The drawing under review shows one solid part. Ordinate dimensions are in mm from its lowest x, y, z. A direction names the side the tool comes from. Coordinates: 2 decimals unless noted, no trailing zeros. Order: outer loops, then holes, each group sorted by start corner. A loop starts at its lowest first (then second) coordinate and runs counter-clockwise, first axis right, second up. Notation, with made-up numbers: M 47.25,14.5 L 100.25,14.5 A22 cw 100.25,34.5 Z; hole C 20.25,-27.5 d4. An arc over 180 degrees is marked long. Answer as a JSON object with one key per item and string values.
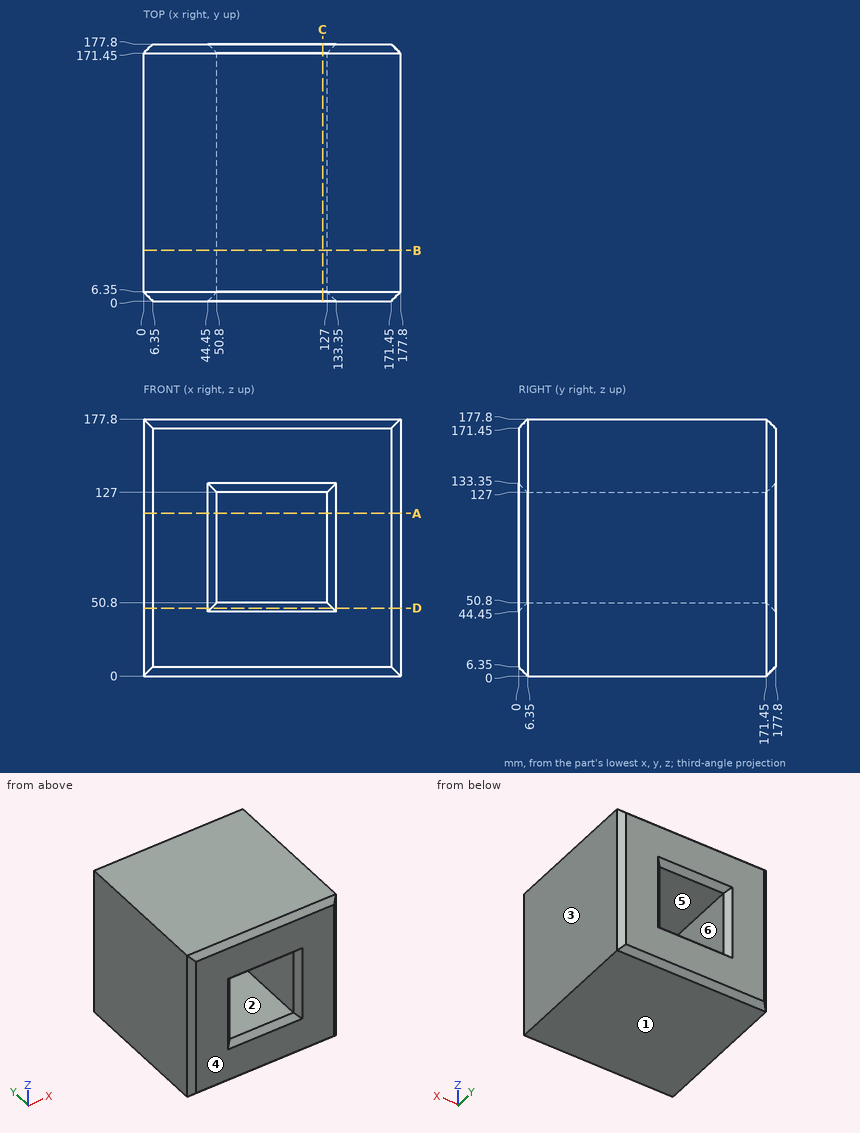
1) Add section D-D (z = 47). State the section outline as (x, y) points, and give its area (3 significant figures).
Taken from the geometry:
{"outline": "M 0,6.35 L 6.35,0 L 44.45,0 L 47,2.55 L 130.8,2.55 L 133.35,0 L 171.45,0 L 177.8,6.35 L 177.8,171.45 L 171.45,177.8 L 133.35,177.8 L 130.8,175.25 L 47,175.25 L 44.45,177.8 L 6.35,177.8 L 0,171.45 Z", "area": "31,100 mm2"}
2) Add section B-B (y = 35). State the section outline as (x, z) points, and give its area (3 significant figures).
Taken from the geometry:
{"outline": "M 0,0 L 177.8,0 L 177.8,177.8 L 0,177.8 Z; hole M 50.8,50.8 L 127,50.8 L 127,127 L 50.8,127 Z", "area": "25,800 mm2"}
3) To check wall thickness, follow L1, parallel to X at y = 89.5, z = 60.5; L2, parallel to Y at x = 46, z = 51. State the ranges of each line that lie inside material, in increasing order.
Taken from the geometry:
{"L1": "x = 0 to 50.8, 127 to 177.8", "L2": "y = 1.55 to 176.25"}
4) Insertion check: pin 1 Ø2 at (x, z) = (66, 127.5) entering from -Y; pin 2 Ø3 at (x, z) = (117, 130) entering from +Y. Each pin has a flat end and moves straight along its axis. Give the tip position at first contact, or say it passes through.
Taken from the geometry:
{"pin 1": "stops at y = 4.85", "pin 2": "stops at y = 175.95"}
5) Add section A-A (z = 112.5). State the section outline as (x, y) points, and give its area (3 significant figures).
Taken from the geometry:
{"outline": "M 0,6.35 L 6.35,0 L 44.45,0 L 50.8,6.35 L 50.8,171.45 L 44.45,177.8 L 6.35,177.8 L 0,171.45 Z; M 127,6.35 L 133.35,0 L 171.45,0 L 177.8,6.35 L 177.8,171.45 L 171.45,177.8 L 133.35,177.8 L 127,171.45 Z", "area": "17,900 mm2"}
6) Tool access review of the marked faces 1 and 2: name each direction out of +Z, -Z, +X, -X, +Y, -Y from which nothing blocks a thin tool from reaching the whole face with its end or side.
Taken from the geometry:
{"face 1": "-Z, +X, -X, +Y, -Y", "face 2": "+Y, -Y"}
7) Mouldability with a two-part tool opening along X and no side actions: class the marked faces 3, 4, 5 and 6 as released by +X, released by -X, zero draft, split by the parting line, or undercut.
Taken from the geometry:
{"face 3": "released by +X", "face 4": "zero draft", "face 5": "undercut", "face 6": "undercut"}
8) Add section C-C (x = 124). State the section outline as (y, z) points.
Taken from the geometry:
{"outline": "M 0,6.35 L 6.35,0 L 171.45,0 L 177.8,6.35 L 177.8,44.45 L 171.45,50.8 L 6.35,50.8 L 0,44.45 Z; M 0,133.35 L 6.35,127 L 171.45,127 L 177.8,133.35 L 177.8,171.45 L 171.45,177.8 L 6.35,177.8 L 0,171.45 Z"}
